Verification items for the finished model (mm, model axes). Give positions to 0.01 mm unless a question says otherwise; leave off trailing zeros.
from build123d import *

# Parameters (mm, degrees)
CROQUIS2_W              = 40
CROQUIS2_H              = 104.5
SALIENTE_EXTRUIR1_DEPTH = 3
CROQUIS3_W              = 3.2
CROQUIS3_H              = 5
CORTAR_EXTRUIR1_DEPTH   = 4
CROQUIS4_R              = 1.5
CORTAR_EXTRUIR3_DEPTH   = 3
CORTAR_EXTRUIR4_DEPTH   = 4


with BuildPart() as part:
    # Croquis2 → Saliente-Extruir1 (new body)
    with BuildSketch(Plane.XY):
        Rectangle(CROQUIS2_W, CROQUIS2_H)
    extrude(amount=SALIENTE_EXTRUIR1_DEPTH)

    # Croquis3 → Cortar-Extruir1 (cut, through all)
    with BuildSketch(Plane.XY.offset(3)):
        with Locations((15.6, 18.75)):
            Rectangle(CROQUIS3_W, CROQUIS3_H)
        with Locations((15.6, 0)):
            Rectangle(CROQUIS3_W, CROQUIS3_H)
        with Locations((15.6, -18.75)):
            Rectangle(CROQUIS3_W, CROQUIS3_H)
        with Locations((-15.6, 18.75)):
            Rectangle(CROQUIS3_W, CROQUIS3_H)
        with Locations((-15.6, 0)):
            Rectangle(CROQUIS3_W, CROQUIS3_H)
        with Locations((-15.6, -18.75)):
            Rectangle(CROQUIS3_W, CROQUIS3_H)
    extrude(amount=-CORTAR_EXTRUIR1_DEPTH, mode=Mode.SUBTRACT)

    # Croquis4 → Cortar-Extruir3 (cut)
    with BuildSketch(Plane.XY.offset(3)):
        with Locations((15.060660172, 20.189339828)):
            Circle(CROQUIS4_R)
        with Locations((16.139339828, 20.189339828)):
            Circle(CROQUIS4_R)
        with Locations((16.139339828, 17.310660172)):
            Circle(CROQUIS4_R)
        with Locations((15.060660172, 17.310660172)):
            Circle(CROQUIS4_R)
    extrude(amount=-CORTAR_EXTRUIR3_DEPTH, mode=Mode.SUBTRACT)

    # Croquis5 → Cortar-Extruir4 (cut, through all)
    with BuildSketch(Plane.XY.offset(3)):
        with BuildLine():
            Line((17.2, 0.378679656), (17.2, -0.378679656))
            ThreePointArc((17.2, -0.378679656), (17.396823775, -2.257101482), (15.6, -2.839022846))
            ThreePointArc((15.6, -2.839022846), (13.803176225, -2.257101482), (14, -0.378679656))
            Line((14, -0.378679656), (14, 0.378679656))
            ThreePointArc((14, 0.378679656), (13.803176225, 2.257101482), (15.6, 2.839022846))
            ThreePointArc((15.6, 2.839022846), (17.396823775, 2.257101482), (17.2, 0.378679656))
        make_face()
        with BuildLine():
            Line((14, -18.371320344), (14, -19.128679656))
            ThreePointArc((14, -19.128679656), (13.803176225, -21.007101482), (15.6, -21.589022846))
            ThreePointArc((15.6, -21.589022846), (17.396823775, -21.007101482), (17.2, -19.128679656))
            Line((17.2, -19.128679656), (17.2, -18.371320344))
            ThreePointArc((17.2, -18.371320344), (17.396823775, -16.492898518), (15.6, -15.910977154))
            ThreePointArc((15.6, -15.910977154), (13.803176225, -16.492898518), (14, -18.371320344))
        make_face()
        with BuildLine():
            Line((-17.2, -19.128679656), (-17.2, -18.371320344))
            ThreePointArc((-17.2, -18.371320344), (-17.396823775, -16.492898518), (-15.6, -15.910977154))
            ThreePointArc((-15.6, -15.910977154), (-13.803176225, -16.492898518), (-14, -18.371320344))
            Line((-14, -18.371320344), (-14, -19.128679656))
            ThreePointArc((-14, -19.128679656), (-13.803176225, -21.007101482), (-15.6, -21.589022846))
            ThreePointArc((-15.6, -21.589022846), (-17.396823775, -21.007101482), (-17.2, -19.128679656))
        make_face()
        with BuildLine():
            Line((-14, -0.378679656), (-14, 0.378679656))
            ThreePointArc((-14, 0.378679656), (-13.803176225, 2.257101482), (-15.6, 2.839022846))
            ThreePointArc((-15.6, 2.839022846), (-17.396823775, 2.257101482), (-17.2, 0.378679656))
            Line((-17.2, 0.378679656), (-17.2, -0.378679656))
            ThreePointArc((-17.2, -0.378679656), (-17.396823775, -2.257101482), (-15.6, -2.839022846))
            ThreePointArc((-15.6, -2.839022846), (-13.803176225, -2.257101482), (-14, -0.378679656))
        make_face()
        with BuildLine():
            Line((-17.2, 18.371320344), (-17.2, 19.128679656))
            ThreePointArc((-17.2, 19.128679656), (-17.396823775, 21.007101482), (-15.6, 21.589022846))
            ThreePointArc((-15.6, 21.589022846), (-13.803176225, 21.007101482), (-14, 19.128679656))
            Line((-14, 19.128679656), (-14, 18.371320344))
            ThreePointArc((-14, 18.371320344), (-13.803176225, 16.492898518), (-15.6, 15.910977154))
            ThreePointArc((-15.6, 15.910977154), (-17.396823775, 16.492898518), (-17.2, 18.371320344))
        make_face()
    extrude(amount=-CORTAR_EXTRUIR4_DEPTH, mode=Mode.SUBTRACT)


solid = part.part
(1) Scan lines: line 1 (Y direction, x = -15, z = 0.95); line 2 (X direction, y = -1.5, z = 1.7); line 3 (X direction, y = 2.5, z = 2.05). Record each from-to range of solid material in increasing order.
Solved:
line 1: y = -52.25 to -21.69, -15.81 to -2.94, 2.94 to 15.81, 21.69 to 52.25
line 2: x = -20 to -17.64, -13.56 to 13.56, 17.64 to 20
line 3: x = -20 to -17.2, -14 to 14, 17.2 to 20
(2) Release check for a two-part mould opening along Y. For faces 1 (the cylindrical face through (17.4, -16.5, 1.5)), 2 (the flat face through (0, 52.25, 1)), 3 (the flat face through (0, 1, 3)) record: pulls with the +Y half, pulls with the -Y half, needs draft (parallel to the pull), parting line crosses it, or undercut.
Solved:
face 1: undercut
face 2: pulls with the +Y half
face 3: needs draft
(3) Section check A-A, the plane z = 1.8. Give the number of separate pieces and of enclosed holes in the cut face, then the cut area to 3 significant figures.
Solved:
separate pieces: 1
enclosed holes: 6
area: 4,060 mm2
(4) Go/stop test with a flat-tipped pin: pin 1 (12 mm diameter, centred on x = 1, y = -5, fed in from -Z). Record where the tip stops, or that it passes through.
Solved:
pin 1: stops at z = 0
